CAD build for the part. Positions are in the model's coordinates, mm. Face numbers are marked on the shaded views. A direction names the side the tool comes from. Give positions to 0.01 mm unless a question says otherwise; leave off trailing zeros. Write each loop counter-clockwise with the first axis right and the second up, starting at its lowest first coordinate (ties: lowest second). Pieces come first, ordered by that corner, then holes. Notation, with made-up numbers: (67, 45.25) -> (105, 45.25) arc R22 cw to (105, 54.25) -> close; hole circle Ø8 at (-11.5, 81.5). An arc over 180 degrees is marked (long way). Answer in a Markdown table with one row per item. Add a question column.
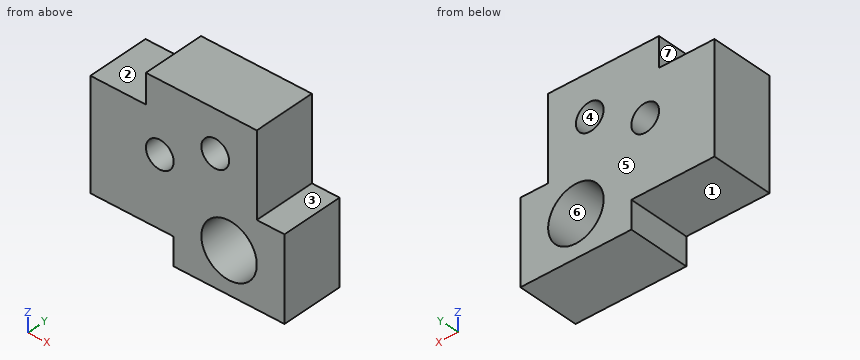
Autodesk Inventor part; units mm, degrees
ref_plane "YZ Plane" through (0, 0, 0) normal (1, 0, 0) x (0, 1, 0)
ref_plane "XZ Plane" through (0, 0, 0) normal (0, 1, 0) x (-1, 0, 0)
ref_plane "XY Plane" through (0, 0, 0) normal (0, 0, 1) x (1, 0, 0)
sketch "Sketch1" plane through (0, 0, 0) normal (0, 1, 0) x (-1, 0, 0)
  line L0 (0, 0) -> (0, 38.1)
  line L1 (0, 38.1) -> (12.7, 38.1)
  line L2 (12.7, 38.1) -> (12.7, 76.2)
  line L3 (0, 0) -> (50.8, 0)
  line L4 (50.8, 0) -> (50.8, 12.7)
  line L5 (50.8, 12.7) -> (88.9, 12.7)
  line L6 (88.9, 12.7) -> (88.9, 62.673)
  circle A0 centre (25.4, 19.05) radius 12.7
  circle A1 centre (31.75, 57.15) radius 6.35
  line L7 (12.7, 76.2) -> (63.5, 76.2)
  line L8 (63.5, 76.2) -> (63.5, 62.673)
  line L9 (63.5, 62.673) -> (88.9, 62.673)
  circle A2 centre (57.15, 44.45) radius 6.35
  dimension "d0" = 38.1
  dimension "d1" = 50.8
  dimension "d2" = 25.4
  dimension "d3" = 12.7
  dimension "d4" = 12.7
extrude "Extrusion1" add sketch "Sketch1" along normal blind 28.575
properties part number "P1-4"
Item 1: Slice it at B-B, the plane x = -57.15. List the corners of the cut face in (y, z) (3 decimals).
Item 2: Slice it at C-C, the plane y = 7.5. List the corners of the cut face in (x, z).
Item 3: Which spindle directions (+Z, -Z, +X, -X, +Y, -Y) get a long thin tool onto all of the face, cutting with end or side? Do the marked faces 1, 2, 3 and 4. Say none if no direction does.
Item 4: Slice it at D-D, the plane x = -33. List the corners of the cut face in (y, z) (3 decimals), then the cut area to 3 significant figures.
Item 5: Slice it at A-A, the plane z = 19.05. List the corners of the cut face in (x, y) (3 decimals), then the cut area to 3 significant figures.
Item 6: Mould opens along X. For the marked faces 5, 6 and 7 say: released by +X, released by -X, zero draft, split by the parting line, or undercut.
Item 7: Drop flat-ended pins along their axis: pin 1 Ø5 at (x, z) = (-33.5, 57) entering from -Y; pin 2 Ø14.5 at (x, y) = (-72, 15.5) entering from -Z; pin 3 Ø7 at (y, z) = (19, 70.5) entering from -X; pin 4 Ø14 at (y, z) = (13, 4.5) entering from -X. Give the stop position or say it passes through.
Item 8: Probe L1, parallel to Z at x = -26.5, y = 22.5; L2, parallel to Z at x = -57.15, y = 20; L3, parallel to X at y = 5.25, z = 19. List the from-to ranges inside material, lowest first. Write a range as from..to.
Answer key:
| question | item | result |
|---|---|---|
| 1 | outline | (0, 12.7) -> (28.575, 12.7) -> (28.575, 38.1) -> (0, 38.1) -> close; (0, 50.8) -> (28.575, 50.8) -> (28.575, 76.2) -> (0, 76.2) -> close |
| 2 | outline | (-88.9, 12.7) -> (-50.8, 12.7) -> (-50.8, 0) -> (0, 0) -> (0, 38.1) -> (-12.7, 38.1) -> (-12.7, 76.2) -> (-63.5, 76.2) -> (-63.5, 62.67) -> (-88.9, 62.67) -> close; hole circle Ø12.7 at (-57.15, 44.45); hole circle Ø25.4 at (-25.4, 19.05); hole circle Ø12.7 at (-31.75, 57.15) |
| 3 | face 1 | -Z, -X, +Y, -Y |
| 3 | face 2 | +Z, -X, +Y, -Y |
| 3 | face 3 | +Z, +X, +Y, -Y |
| 3 | face 4 | +Y, -Y |
| 4 | outline | (0, 0) -> (28.575, 0) -> (28.575, 8.875) -> (0, 8.875) -> close; (0, 29.225) -> (28.575, 29.225) -> (28.575, 50.924) -> (0, 50.924) -> close; (0, 63.376) -> (28.575, 63.376) -> (28.575, 76.2) -> (0, 76.2) -> close |
| 4 | area | 1,240 mm² |
| 5 | outline | (-88.9, 0) -> (-38.1, 0) -> (-38.1, 28.575) -> (-88.9, 28.575) -> close; (-12.7, 0) -> (0, 0) -> (0, 28.575) -> (-12.7, 28.575) -> close |
| 5 | area | 1,810 mm² |
| 6 | face 5 | zero draft |
| 6 | face 6 | undercut |
| 6 | face 7 | released by -X |
| 7 | pin 1 | passes through |
| 7 | pin 2 | stops at z = 12.7 |
| 7 | pin 3 | stops at x = -63.5 |
| 7 | pin 4 | stops at x = -50.8 |
| 8 | L1 | z = 0..6.4, 31.7..53.58, 60.72..76.2 |
| 8 | L2 | z = 12.7..38.1, 50.8..76.2 |
| 8 | L3 | x = -88.9..-38.1, -12.7..0 |
